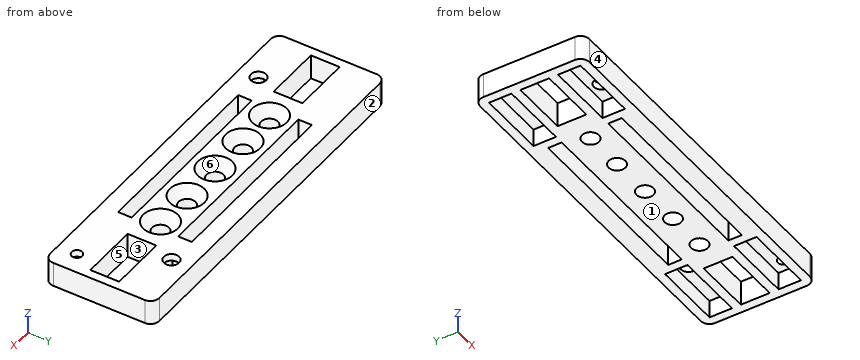
```python
from build123d import *

# Parameters (mm, degrees)
F0_W           = 81.1
F0_H           = 24.65
F1_DEPTH       = 5.6
F3_D           = 3.45
F4_D           = 2.39
F6_D           = 3.7973
F6_CSINK_D     = 7.7978
F6_CSINK_ANGLE = 82
F7_R           = 1.725
F7_R_2         = 1.195
F8_DEPTH       = 3.9998
F7_W           = 42
F7_H           = 3.075
F7_W_2         = 13
F7_H_2         = 6.5
F9_DEPTH       = 5.6
F10_R          = 2


# Not quite as in the source:
# - a feature names something its author has since deleted; it is built from what else it names


with BuildPart() as f1:
    # F0 (on Top) → F1 (new body)
    with BuildSketch(Plane.XY):
        Rectangle(F0_W, F0_H)
    extrude(amount=F1_DEPTH)

    # F3 (through all)
    with Locations(Plane.XY.offset(5.6)):
        with Locations((-27.6, -8), (27.6, 8)):
            Hole(F3_D / 2)

    # F4 (through all)
    with Locations(Plane.XY.offset(5.6)):
        with Locations((35.88, -8)):
            Hole(F4_D / 2)

    # F6 (through all)
    with Locations(Plane.XY.offset(5.6)):
        with Locations((-19.05, 0), (-9.779, 0), (0, 0), (9.779, 0), (19.05, 0)):
            CounterSinkHole(F6_D / 2, F6_CSINK_D / 2, counter_sink_angle=F6_CSINK_ANGLE)

    # F7 (on face) → F8 (cut, through all)
    with BuildSketch(Plane(origin=(0, 0, 0), x_dir=(1, 0, 0), z_dir=(0, 0, -1))):
        Polygon((-38.55, 10.325), (-38.55, 5.25), (-23.55, 5.25), (-23, 5.25), (-23, 10.325), align=None)
        with Locations((-27.6, 8)):
            Circle(F7_R, mode=Mode.SUBTRACT)
        Polygon((-23.55, -5.25), (-38.55, -5.25), (-38.55, -10.325), (-23, -10.325), (-23, -5.25), align=None)
        Polygon((38.55, -10.325), (38.55, -5.25), (23.55, -5.25), (23, -5.25), (23, -10.325), align=None)
        with Locations((27.6, -8)):
            Circle(F7_R, mode=Mode.SUBTRACT)
        Polygon((23.55, 5.25), (38.55, 5.25), (38.55, 10.325), (23, 10.325), (23, 5.25), align=None)
        with Locations((35.88, 8)):
            Circle(F7_R_2, mode=Mode.SUBTRACT)
    extrude(amount=-F8_DEPTH, mode=Mode.SUBTRACT)

    # F7 (on face) → F9 (cut, through all)
    with BuildSketch(Plane(origin=(0, 0, 0), x_dir=(1, 0, 0), z_dir=(0, 0, -1))):
        with Locations((0, -6.7875)):
            Rectangle(F7_W, F7_H)
        with Locations((-32.05, 0)):
            Rectangle(F7_W_2, F7_H_2)
        with Locations((32.05, 0)):
            Rectangle(F7_W_2, F7_H_2)
        with Locations((0, 6.7875)):
            Rectangle(F7_W, F7_H)
    extrude(amount=-F9_DEPTH, mode=Mode.SUBTRACT)

    # F10
    f10_edges = [f1.edges().sort_by_distance(p)[0] for p in [
        (40.55, 12.325, 2.8),
        (-40.55, 12.325, 2.8),
        (-40.55, -12.325, 2.8),
        (40.55, -12.325, 2.8),
    ]]
    fillet(f10_edges, radius=F10_R)


solid = f1.part
```
Work out the finished part from the listing and answer in its coordinate system (mm). Face numbers are marked on the shaded views. A direction names the side the tool comes from. Round coordinates to 2 decimals unless told otherwise and drop trailing zeros. Loops run counter-clockwise (first coordinate to the right, second up) from the corner with the lowest first, then second, coordinate; pieces in that order, holes last.
(1) The part is cut by section B-B, the plane y = 0. Give the number of separate pieces and of enclosed holes in the cut face, and give its area (3 significant figures).
Computed values:
separate pieces: 8
enclosed holes: 0
area: 179 mm2
(2) Find the intervals of material crossed by L1, parallel to X at y = 3, z = 1; L2, parallel to X at y = -5.75, z = 3.05; L3, parallel to Y at x = -16, z = 3.3 (3 decimals), in increasing order.
Computed values:
L1: x = -40.55 to -38.55, -25.55 to 25.55, 38.55 to 40.55
L2: x = -40.55 to -38.55, -23 to -21, 21 to 23, 38.55 to 40.55
L3: y = -12.325 to -8.325, -5.25 to 5.25, 8.325 to 12.325
(3) For the marked faces 5 and 6, determine the directions among +Z, -Z, +X, -X, +Y, -Y from which every point of the face is accessible in a straight line to the end or side of a thin tool.
Computed values:
face 5: +Z, -Z
face 6: +Z
(4) The part is cut by section A-A, the plane x = 35.88. Give the vertices of the cut face in (y, z) (3 decimals), and give its area (3 significant figures).
Computed values:
outline: (-12.325, 0) - (-10.325, 0) - (-10.325, 4) - (-9.195, 4) - (-9.195, 5.6) - (-12.325, 5.6) - close; (-6.805, 4) - (-5.25, 4) - (-5.25, 0) - (-3.25, 0) - (-3.25, 5.6) - (-6.805, 5.6) - close; (3.25, 0) - (5.25, 0) - (5.25, 4) - (10.325, 4) - (10.325, 0) - (12.325, 0) - (12.325, 5.6) - (3.25, 5.6) - close
area: 57.2 mm2
(5) The mould has two halves that part along Y. Classify the marked faces 1, 2, 3 and 4: pulls with the +Y half, pulls with the -Y half, needs draft (parallel to the pull), parting line crosses it, or undercut.
Computed values:
face 1: needs draft
face 2: pulls with the +Y half
face 3: undercut
face 4: pulls with the -Y half
(6) This flat-tipped pin is pushed along its axis until it touches: P1, Ø6, axis at x = 0, y = 0, coming from the +Z side. Where does it stop, or does it pass through?
Computed values:
P1: stops at z = 4.57
(7) The part is cut by section C-C, the plane x = -27.6. Give the vertices of the cut face in (y, z) (3 decimals), and give its area (3 significant figures).
Computed values:
outline: (-12.325, 0) - (-10.325, 0) - (-10.325, 4) - (-9.725, 4) - (-9.725, 5.6) - (-12.325, 5.6) - close; (-6.275, 4) - (-5.25, 4) - (-5.25, 0) - (-3.25, 0) - (-3.25, 5.6) - (-6.275, 5.6) - close; (3.25, 0) - (5.25, 0) - (5.25, 4) - (10.325, 4) - (10.325, 0) - (12.325, 0) - (12.325, 5.6) - (3.25, 5.6) - close
area: 55.5 mm2
